Build history of the part. All positions in model axes, mm. A direction names the side the tool comes from. Give positions to 0.01 mm unless a question says otherwise; leave off trailing zeros. Order: outer loops, then holes, each group sorted by start corner. A loop starts at its lowest first (then second) coordinate and runs counter-clockwise, first axis right, second up. Notation, with made-up numbers: (-17, -24) - (41, -24) arc R18 cw to (41, -4) - close; hole circle Ø8 at (53, -39). An arc over 180 degrees is marked (long way). One line per item, written item: value.
```python
from build123d import *

# Parameters (mm, degrees)
F1_DEPTH = 11
F2_W     = 4.5
F2_H     = 6
F3_DEPTH = 5
F4_W     = 3
F4_H     = 7
F5_DEPTH = 8.501
F6_W     = 4.5
F6_H     = 6
F7_DEPTH = 5
F8_W     = 3.5
F8_H     = 7
F9_DEPTH = 8.501


with BuildPart() as f1:
    # F0 (on Top) → F1 (new body)
    with BuildSketch(Plane.XY):
        Polygon((0, -8.5), (0, 0), (-19.8, 0), (-19.8, -8.5), (-14.8, -8.5), (-14.8, -11), (-12.3, -11), (-12.3, -2.5), (-10, -2.5), (-10, -11), (-7.5, -11), (-7.5, -8.5), align=None)
    extrude(amount=F1_DEPTH)

    # F2 (on face) → F3 (cut, through all)
    with BuildSketch(Plane(origin=(-19.8, 0, 0), x_dir=(0, -1, 0), z_dir=(-1, 0, 0))):
        with Locations((4.25, 6)):
            Rectangle(F2_W, F2_H)
    extrude(amount=-F3_DEPTH, mode=Mode.SUBTRACT)

    # F4 (on face) → F5 (cut, through all)
    with BuildSketch(Plane.XZ.offset(8.5)):
        with Locations((-16.3, 5.5)):
            Rectangle(F4_W, F4_H)
    extrude(amount=-F5_DEPTH, mode=Mode.SUBTRACT)

    # F6 (on face) → F7 (cut)
    with BuildSketch(Plane.YZ):
        with Locations((-4.25, 6)):
            Rectangle(F6_W, F6_H)
    extrude(amount=-F7_DEPTH, mode=Mode.SUBTRACT)

    # F8 (on face) → F9 (cut, through all)
    with BuildSketch(Plane.XZ.offset(8.5)):
        with Locations((-3.75, 5.5)):
            Rectangle(F8_W, F8_H)
    extrude(amount=-F9_DEPTH, mode=Mode.SUBTRACT)


solid = f1.part
```
(1) 3-axis set-ups, long thin cutter, end or side, ignore diameter. For faces 4 (the face through (-17, -4, 9)), 5 (the face through (-5.5, -4, 5)), 6 (the face through (-11, -2.5, 5)), 7 (the face through (-19, -2, 6)), 8 (the face through (-14.8, -7, 5)): which of +Z, -Z, +X, -X, +Y, -Y reach the whole face in a straight line?
Completed:
face 4: none
face 5: +Y, -Y
face 6: +Z, -Z, -Y
face 7: -X
face 8: -Y
(2) Slice it at D-D, the plane y = -7.5. Give the cut face in (x, z), and give its area (3 significant figures).
Completed:
outline: (-19.8, 0) - (-12.3, 0) - (-12.3, 11) - (-19.8, 11) - close; (-10, 0) - (0, 0) - (0, 11) - (-10, 11) - close; hole (-17.8, 2) - (-14.8, 2) - (-14.8, 9) - (-17.8, 9) - close; hole (-5.5, 2) - (-2, 2) - (-2, 9) - (-5.5, 9) - close
area: 147 mm²
(3) Pin check, flat tips, straight feed: P1, Ø1.5, axis at x = -18, z = 4, coming from the -Y side; P2, Ø2, axis at y = -10, z = 5.5, coming from the +X side. Stop position of each tip, or through.
Completed:
P1: y = -8.5
P2: x = -7.5
(4) Pull direction X, two halves, no side cores. Call faces 1 (the face through (-12.3, -7, 5)), 2 (the face through (-19, -6.5, 6)), 3 (the face through (-7.5, -10, 5)): +X half, -X half, draft (parallel to the pull), parting line (faces both ways), or undercut.
Completed:
face 1: undercut
face 2: draft
face 3: +X half
(5) Slice it at C-C, the plane x = -3.75. Give the cut face in (y, z).
Completed:
outline: (-8.5, 0) - (0, 0) - (0, 2) - (-8.5, 2) - close; (-8.5, 9) - (0, 9) - (0, 11) - (-8.5, 11) - close
(6) Slice it at B-B, the plane y = -6. Give the cut face in (x, z), and give its area (3 significant figures).
Completed:
outline: (-19.8, 0) - (-12.3, 0) - (-12.3, 11) - (-19.8, 11) - (-19.8, 9) - (-14.8, 9) - (-14.8, 2) - (-17.8, 2) - (-17.8, 3) - (-19.8, 3) - close; (-10, 0) - (0, 0) - (0, 3) - (-2, 3) - (-2, 2) - (-5.5, 2) - (-5.5, 9) - (0, 9) - (0, 11) - (-10, 11) - close
area: 123 mm²
(7) Drill centre lines: line 1 (X direction, y = -1.25, z = 4.5); line 2 (Y direction, x = -18, z = 6.75); line 3 (X direction, y = -4, z = 7). Where is each one in solid material? Low to high.
Completed:
line 1: -19.8 to -17.8, -14.8 to -5.5, -2 to 0
line 2: -8.5 to -6.5, -2 to 0
line 3: -14.8 to -12.3, -10 to -5.5
(8) Slice it at A-A, the plane z = 6.5. Give the cut face in (x, y), and give its area (4 significant figures).
Completed:
outline: (-19.8, -8.5) - (-17.8, -8.5) - (-17.8, -6.5) - (-19.8, -6.5) - close; (-19.8, -2) - (-17.8, -2) - (-17.8, 0) - (-19.8, 0) - close; (-14.8, -11) - (-12.3, -11) - (-12.3, -2.5) - (-10, -2.5) - (-10, -11) - (-7.5, -11) - (-7.5, -8.5) - (-5.5, -8.5) - (-5.5, 0) - (-14.8, 0) - close; (-2, -8.5) - (0, -8.5) - (0, -6.5) - (-2, -6.5) - close; (-2, -2) - (0, -2) - (0, 0) - (-2, 0) - close
area: 93.75 mm²
